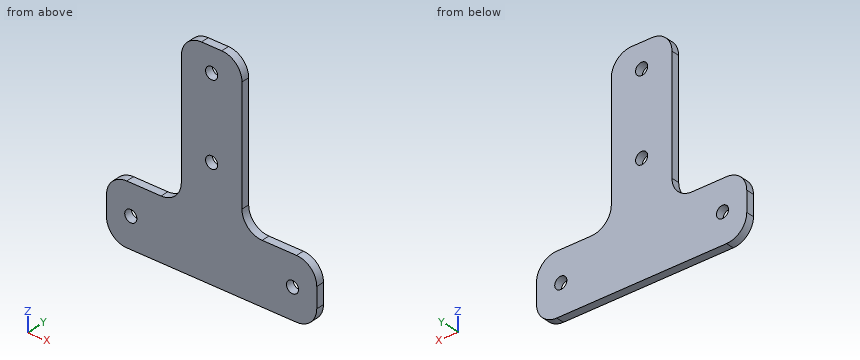
from build123d import *

# Parameters (mm, degrees)
SKETCH1_R           = 1.5
BOSS_EXTRUDE1_DEPTH = 2
FILLET1_R           = 5


with BuildPart() as part:
    # Sketch1 → Boss-Extrude1 (new body)
    with BuildSketch(Plane(origin=(0, 0, 0), x_dir=(1, 0, 0), z_dir=(0, 1, 0))):
        Polygon((7.5, -46), (7.5, -7.5), (26, -7.5), (26, 7.5), (-26, 7.5), (-26, -7.5), (-7.5, -7.5), (-7.5, -46), align=None)
        with Locations((0, -40)):
            Circle(SKETCH1_R, mode=Mode.SUBTRACT)
        with Locations((0, -20)):
            Circle(SKETCH1_R, mode=Mode.SUBTRACT)
        with Locations((20, 0)):
            Circle(SKETCH1_R, mode=Mode.SUBTRACT)
        with Locations((-20, 0)):
            Circle(SKETCH1_R, mode=Mode.SUBTRACT)
    extrude(amount=BOSS_EXTRUDE1_DEPTH)

    # Fillet1
    fillet1_edges = [part.edges().sort_by_distance(p)[0] for p in [
        (-7.5, 1, 46),
        (-7.5, 1, 7.5),
        (-26, 1, 7.5),
        (-26, 1, -7.5),
        (26, 1, -7.5),
        (26, 1, 7.5),
        (7.5, 1, 7.5),
        (7.5, 1, 46),
    ]]
    fillet(fillet1_edges, radius=FILLET1_R)


solid = part.part
Can you work these out from the model? Positions are in its coordinate system, mm. Coordinates: 2 decimals unless noted, no trailing zeros. Order: outer loops, then holes, each group sorted by start corner. A loop starts at its lowest first (then second) coordinate and runs counter-clockwise, first axis right, second up. Notation, with made-up numbers: M 4,-2.5 L 11,-2.5 A23 ccw 11,33.5 Z; hole C 86.5,51.5 d8. An arc over 180 degrees is marked long. Write item = value, one per line.
(1) Suppose I cut it at B-B on z = 0. Please give me the cut outline in (x, y).
Results are:
outline = M -26,0 L -21.5,0 L -21.5,2 L -26,2 Z; M -18.5,0 L 18.5,0 L 18.5,2 L -18.5,2 Z; M 21.5,0 L 26,0 L 26,2 L 21.5,2 Z
(2) Suppose I cut it at D-D on y = 0.5. Please give me the cut outline in (x, z), plus the area to 3 significant figures.
Results are:
outline = M -26,-2.5 A5 ccw -21,-7.5 L 21,-7.5 A5 ccw 26,-2.5 L 26,2.5 A5 ccw 21,7.5 L 12.5,7.5 A5 cw 7.5,12.5 L 7.5,41 A5 ccw 2.5,46 L -2.5,46 A5 ccw -7.5,41 L -7.5,12.5 A5 cw -12.5,7.5 L -21,7.5 A5 ccw -26,2.5 Z; hole C -20,0 d3; hole C 0,20 d3; hole C 0,40 d3; hole C 20,0 d3
area = 1,310 mm2
(3) For pin 1 Ø0.6 at (y, z) = (1.5, 20) entering from -X, with a flat end and sliding along its axis, tell me the tip position at first contact or that it passes through.
Results are:
pin_1 = -7.5
(4) Suppose I cut it at C-C on z = 40. Please give me the cut outline in (x, y), plus the area to 3 significant figures.
Results are:
outline = M -7.5,0 L -1.5,0 L -1.5,2 L -7.5,2 Z; M 1.5,0 L 7.5,0 L 7.5,2 L 1.5,2 Z
area = 24.0 mm2
(5) I need wall thicknesses on line 1 along Z through (x, y) = (0, 1.5); line 2 along X through (y, z) = (1.15, 0); line 3 along X through (y, z) = (0.9, 20). Which ranges of each line are inside material? Lowest first, please. Write a range as [from, to].
Results are:
line_1 = [-7.5, 18.5], [21.5, 38.5], [41.5, 46]
line_2 = [-26, -21.5], [-18.5, 18.5], [21.5, 26]
line_3 = [-7.5, -1.5], [1.5, 7.5]
(6) Suppose I cut it at A-A on x = 0. Please give me the cut outline in (y, z).
Results are:
outline = M 0,-7.5 L 2,-7.5 L 2,18.5 L 0,18.5 Z; M 0,21.5 L 2,21.5 L 2,38.5 L 0,38.5 Z; M 0,41.5 L 2,41.5 L 2,46 L 0,46 Z
